Geometry: final body of the model. Coordinates: model frame, mm. Coordinates: 2 decimals unless noted, no trailing zeros. Order: outer loops, then holes, each group sorted by start corner. A loop starts at its lowest first (then second) coordinate and runs counter-clockwise, first axis right, second up. Notation, with made-up numbers: (32.5, -21) -> (81.5, -21) arc R31 ccw to (81.5, 9) -> close; hole circle Ø7 at (-38.5, 48). An arc over 180 degrees is marked (long way). Answer in a Markdown table with one row per item. Add a question column.
1) Ray query, line 1 (Z direction, x = 11.75, y = -1.75); line 2 (Y direction, x = 14, z = -1.3); line 3 (X direction, y = 0.5, z = -1.85). Return the intervals inside material, ascending. Write a range as from..to.
2) Section query A-A on x = 11.25. Return the cut outline in (y, z), then the cut area to 3 significant figures.
3) Section query D-D on y = 2.75. Return the cut outline in (x, z).
4) Section query C-C on y = -2. Return the cut outline in (x, z), then the cut area to 3 significant figures.
5) Contact query for flat-ended pins moving along their axis: P1, Ø1, axis at y = 3.5, z = -0.5, coming from the -X side; P2, Ø0.8, axis at x = 11.5, y = -2, coming from the -Z side; P3, Ø1.3, axis at y = -0.5, z = 0.5, coming from the +X side; P4, Ø0.5, axis at x = 9.5, y = 2, coming from the +Z side. Output: stop coordinate, or through.
6) Section query B-B on z = 1.1. Return the cut outline in (x, y).
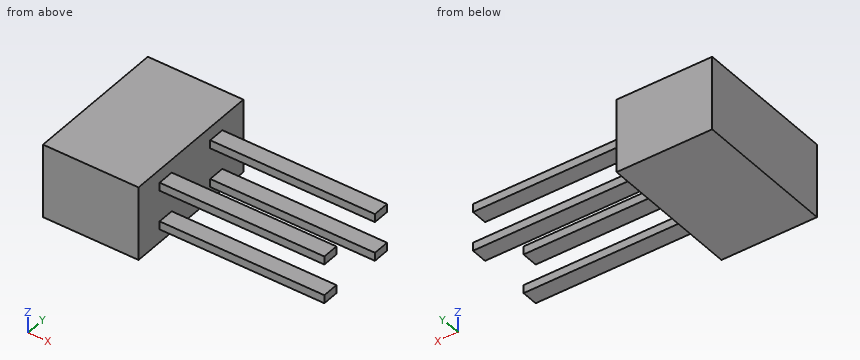
```python
from build123d import *

# Parameters (mm, degrees)
SKETCH1_W           = 4.5
SKETCH1_H           = 8.7
BOSS_EXTRUDE1_DEPTH = 5.8
SKETCH2_W           = 0.5
SKETCH2_H           = 1
BOSS_EXTRUDE2_DEPTH = 10


with BuildPart() as part:
    # Sketch1 → Boss-Extrude1 (new body)
    with BuildSketch(Plane(origin=(0, 0, 0), x_dir=(0, 0, -1), z_dir=(1, 0, 0))):
        Rectangle(SKETCH1_W, SKETCH1_H)
    extrude(amount=BOSS_EXTRUDE1_DEPTH)

    # Sketch2 → Boss-Extrude2 (add)
    with BuildSketch(Plane(origin=(5.8, 0, 0), x_dir=(0, 0, -1), z_dir=(1, 0, 0))):
        with Locations((-1.2, -2.1)):
            Rectangle(SKETCH2_W, SKETCH2_H)
        with Locations((-1.2, 2.1)):
            Rectangle(SKETCH2_W, SKETCH2_H)
        with Locations((1.2, 2.1)):
            Rectangle(SKETCH2_W, SKETCH2_H)
        with Locations((1.2, -2.1)):
            Rectangle(SKETCH2_W, SKETCH2_H)
    extrude(amount=BOSS_EXTRUDE2_DEPTH)


solid = part.part
```
Result:
| question | item | result |
|---|---|---|
| 1 | line 1 | -1.45..-0.95, 0.95..1.45 |
| 1 | line 2 | -2.6..-1.6, 1.6..2.6 |
| 1 | line 3 | 0..5.8 |
| 2 | outline | (-2.6, -1.45) -> (-1.6, -1.45) -> (-1.6, -0.95) -> (-2.6, -0.95) -> close; (-2.6, 0.95) -> (-1.6, 0.95) -> (-1.6, 1.45) -> (-2.6, 1.45) -> close; (1.6, -1.45) -> (2.6, -1.45) -> (2.6, -0.95) -> (1.6, -0.95) -> close; (1.6, 0.95) -> (2.6, 0.95) -> (2.6, 1.45) -> (1.6, 1.45) -> close |
| 2 | area | 2.00 mm2 |
| 3 | outline | (0, -2.25) -> (5.8, -2.25) -> (5.8, 2.25) -> (0, 2.25) -> close |
| 4 | outline | (0, -2.25) -> (5.8, -2.25) -> (5.8, -1.45) -> (15.8, -1.45) -> (15.8, -0.95) -> (5.8, -0.95) -> (5.8, 0.95) -> (15.8, 0.95) -> (15.8, 1.45) -> (5.8, 1.45) -> (5.8, 2.25) -> (0, 2.25) -> close |
| 4 | area | 36.1 mm2 |
| 5 | P1 | x = 0 |
| 5 | P2 | z = -1.45 |
| 5 | P3 | x = 5.8 |
| 5 | P4 | z = 1.45 |
| 6 | outline | (0, -4.35) -> (5.8, -4.35) -> (5.8, -2.6) -> (15.8, -2.6) -> (15.8, -1.6) -> (5.8, -1.6) -> (5.8, 1.6) -> (15.8, 1.6) -> (15.8, 2.6) -> (5.8, 2.6) -> (5.8, 4.35) -> (0, 4.35) -> close |
